CAD build for the part. Positions are in the model's coordinates, mm. A direction names the side the tool comes from. Round coordinates to 2 decimals unless told otherwise and drop trailing zeros. Loops run counter-clockwise (first coordinate to the right, second up) from the corner with the lowest first, then second, coordinate; pieces in that order, holes last.
Autodesk Inventor part; units mm, degrees
ref_plane "Work Plane1" through (-57.15, 3.175, 0) normal (1, 0, 0) x (0, 0, -1)
ref_plane "YZ Plane" through (0, 0, 0) normal (1, 0, 0) x (0, 1, 0)
ref_plane "XZ Plane" through (0, 0, 0) normal (0, 1, 0) x (-1, 0, 0)
sketch "Sketch1" plane through (0, 0, 0) normal (0, 0, 1) x (1, 0, 0)
  line L0 (0, 0) -> (-114.3, 0)
  line L1 (-114.3, 0) -> (-114.3, 63.5)
  line L2 (-114.3, 63.5) -> (0, 63.5)
  line L3 (0, 63.5) -> (0, 0)
  dimension "d7" = 114.3
  dimension "d8" = 63.5
extrude "Extrusion1" add sketch "Sketch1" along normal blind 6.35
sketch "Sketch2" plane through (0, 0, 6.35) normal (0, 0, 1) x (1, 0, 0)
  line L0 (0, 0) -> (0, 63.5)
  line L1 (-114.3, 63.5) -> (-114.3, 0)
  line L2 (-114.3, 0) -> (0, 0)
  line L3 (0, 63.5) -> (-114.3, 63.5)
sketch "Sketch3" plane through (0, 0, 6.35) normal (0, 0, 1) x (1, 0, 0)
  line L0 (-110.6716, 35.2666) -> (-52.0005, 35.2666) construction
  line L1 (-52.0005, 35.2666) -> (-52.0005, 28.3217) construction
  line L2 (-52.0005, 28.3217) -> (-110.6716, 28.3217) construction
  line L3 (-110.6716, 28.3217) -> (-110.6716, 35.2666) construction
  line L4 (-114.3, 63.5) -> (-114.3, 0)
  point P0 (0, 0)
extrude "Extrusion2" [suppressed]
fillet "Fillet2" radius 3.175 4 edges at (-114.3, 63.5, 3.175) (-114.3, 0, 3.175) (0, 0, 3.175) (0, 63.5, 3.175)
sketch "Sketch4" plane through (0, 0, 6.35) normal (0, 0, 1) x (1, 0, 0)
  point P0 (0, 0)
sketch "Sketch5" plane through (0, 0, 6.35) normal (0, 0, 1) x (1, 0, 0)
  point P0 (0, 0)
sketch "Sketch6" plane through (0, 0, 6.35) normal (0, 0, 1) x (1, 0, 0)
  point P0 (0, 0)
ref_plane "Work Plane1" through (-57.15, 3.175, 0) normal (1, 0, 0) x (0, 0, -1)
sketch "Sketch7" plane through (-111.125, 63.5, 0) normal (0, 1, 0) x (1, 0, 0)
  line L0 (107.95, -6.35) -> (0, -6.35)
  line L1 (107.95, 0) -> (0, 0)
  line L2 (0, -6.35) -> (0, -3.175)
  line L3 (0, -6.35) -> (0, 0)
  line L4 (0, 0) -> (0, -6.35)
  line L5 (0, -6.35) -> (0, -3.5306)
  line L6 (0, -3.5306) -> (6.985, -3.5306)
  line L7 (6.985, -3.5306) -> (11.8618, -3.5306)
  line L8 (11.8618, -3.5306) -> (11.8618, -1.651)
  line L9 (11.8618, -1.651) -> (6.985, -1.651)
  line L10 (6.985, -1.651) -> (6.985, -3.5306)
  point P0 (111.125, 0)
  dimension "d24" = 4.8768
  dimension "d25" = 1.8796
  dimension "d26" = 2.8194
  dimension "d27" = 6.985
extrude "Extrusion3" [suppressed]
sketch "Sketch8" plane through (-111.125, 0, 0) normal (0, -1, 0) x (1, 0, 0)
  line L0 (0, 0) -> (0, 6.35)
  line L1 (6.985, 3.5306) -> (6.985, 1.651)
  line L2 (11.8618, 1.651) -> (11.8618, 3.5306)
  line L3 (6.985, 1.651) -> (11.8618, 1.651)
  line L4 (11.8618, 1.651) -> (11.8618, 3.5306)
  line L5 (11.8618, 3.5306) -> (6.985, 3.5306)
  line L6 (6.985, 3.5306) -> (6.985, 1.651)
  line L7 (0, 0) -> (107.95, 0)
  point P0 (111.125, 0)
extrude "Extrusion4" [suppressed]
mirror "Mirror1" [suppressed]
mirror "Mirror2" [suppressed]
sketch "Sketch9" plane through (0, 0, 6.35) normal (0, 0, 1) x (1, 0, 0)
  point P0 (0, 0)
sketch "Sketch10" plane through (0, 0, 6.35) normal (0, 0, 1) x (1, 0, 0)
  line L0 (-111.2518, 27.0157) -> (-111.2518, 30.2464) construction
  line L1 (-111.2518, 30.2464) -> (-93.1484, 30.2464) construction
  line L2 (-93.1484, 30.2464) -> (-93.1484, 27.0157) construction
  line L3 (-93.1484, 27.0157) -> (-111.2518, 27.0157) construction
  line L4 (-114.3, 60.325) -> (-114.3, 3.175)
  line L5 (-114.3, 60.325) -> (-114.3, 3.175)
  line L6 (-114.3, 3.175) -> (-114.3, 31.75)
  line L7 (0, 3.175) -> (0, 60.325)
  line L8 (-88.3918, 11.8288) -> (-102.3042, 15.3115)
  line L9 (-102.3042, 15.3115) -> (-102.3042, 42.6731)
  line L10 (-102.3042, 42.6731) -> (-103.638, 42.988)
  spline S0 degree 2 poles (-103.638, 42.988) (-104.2308, 43.1362) (-105.2867, 42.8213) (-106.0833, 42.1173) (-106.5464, 41.0799) (-106.5464, 40.5242) knots 0 0 0 1 2 3 4 4 4
  line L11 (-106.5464, 40.5242) -> (-106.5464, 12.3845)
  spline S1 degree 2 poles (-106.5464, 12.3845) (-107.4912, 12.8106) (-109.7327, 13.8295) (-110.6775, 14.3297) knots 0 0 0 1 2 2 2
  line L12 (-110.6775, 14.3297) -> (-111.2518, 14.7743)
  line L13 (-111.2518, 14.7743) -> (-111.2518, 45.3222)
  spline S2 degree 2 poles (-111.2518, 45.3222) (-111.2518, 46.5078) (-110.6034, 49.1569) (-109.2881, 51.3984) (-107.38, 52.8434) (-106.0648, 52.8063) knots 0 0 0 1 2 3 4 4 4
  line L14 (-106.0648, 52.8063) -> (-88.3918, 48.3974)
  line L15 (-88.3918, 48.3974) -> (-88.3918, 39.1904)
  line L16 (-88.3918, 39.1904) -> (-97.5988, 41.469)
  line L17 (-97.5988, 41.469) -> (-97.5988, 23.3143)
  line L18 (-97.5988, 23.3143) -> (-88.3918, 21.0358)
  line L19 (-88.3918, 21.0358) -> (-88.3918, 11.8288)
  spline S3 degree 2 poles (-81.1464, 13.144) (-82.0912, 13.5701) (-84.3327, 14.589) (-85.2775, 15.0892) knots 0 0 0 1 2 2 2
  line L20 (-85.2775, 15.0892) -> (-85.8518, 15.5338)
  line L21 (-85.8518, 15.5338) -> (-85.8518, 54.3439)
  spline S4 degree 2 poles (-85.8518, 54.3439) (-84.907, 53.9734) (-82.6655, 52.9175) (-81.7207, 52.3803) knots 0 0 0 1 2 2 2
  line L22 (-81.7207, 52.3803) -> (-81.1464, 51.9357)
  line L23 (-81.1464, 51.9357) -> (-81.1464, 39.0051)
  line L24 (-81.1464, 39.0051) -> (-62.9918, 34.485)
  line L25 (-62.9918, 34.485) -> (-62.9918, 25.278)
  line L26 (-62.9918, 25.278) -> (-81.1464, 29.7981)
  line L27 (-81.1464, 29.7981) -> (-81.1464, 13.144)
  spline S5 degree 2 poles (-42.7788, 11.1619) (-41.4635, 11.1248) (-39.5555, 12.5512) (-38.2402, 14.7928) (-37.5918, 17.4419) (-37.5918, 18.6275) knots 0 0 0 1 2 3 4 4 4
  line L28 (-37.5918, 18.6275) -> (-37.5918, 46.6004)
  line L29 (-37.5918, 46.6004) -> (-60.4518, 52.2876)
  line L30 (-60.4518, 52.2876) -> (-60.4518, 43.0806)
  line L31 (-60.4518, 43.0806) -> (-42.2972, 38.5605)
  line L32 (-42.2972, 38.5605) -> (-42.2972, 23.407)
  spline S6 degree 2 poles (-42.2972, 23.407) (-42.2972, 22.8697) (-42.7603, 21.8509) (-43.5569, 21.1284) (-44.6128, 20.8134) (-45.1871, 20.9431) knots 0 0 0 1 2 3 4 4 4
  line L33 (-45.1871, 20.9431) -> (-60.4518, 24.7593)
  line L34 (-60.4518, 24.7593) -> (-60.4518, 15.5523)
  line L35 (-60.4518, 15.5523) -> (-42.7788, 11.1619)
  line L36 (-35.0518, 12.403) -> (-12.1918, 6.7158)
  line L37 (-12.1918, 6.7158) -> (-12.1918, 15.9228)
  line L38 (-12.1918, 15.9228) -> (-27.475, 19.7205)
  spline S7 degree 2 poles (-27.475, 19.7205) (-26.5302, 20.7393) (-24.1775, 22.9809) (-21.5655, 25.3336) (-18.8238, 27.6863) (-17.4715, 28.8534) knots 0 0 0 1 2 3 4 4 4
  line L39 (-17.4715, 28.8534) -> (-17.4715, 28.9645)
  spline S8 degree 2 poles (-17.4715, 28.9645) (-18.8238, 30.78) (-21.6026, 34.5406) (-24.2146, 38.1715) (-26.5302, 41.5986) (-27.475, 43.0992) knots 0 0 0 1 2 3 4 4 4
  line L40 (-27.475, 43.0992) -> (-12.1918, 39.283)
  line L41 (-12.1918, 39.283) -> (-12.1918, 48.49)
  line L42 (-12.1918, 48.49) -> (-35.0518, 54.1772)
  line L43 (-35.0518, 54.1772) -> (-35.0518, 44.2107)
  spline S9 degree 2 poles (-35.0518, 44.2107) (-34.5146, 43.0621) (-33.014, 40.376) (-31.2171, 37.5046) (-29.2164, 34.5406) (-28.1975, 33.0215) knots 0 0 0 1 2 3 4 4 4
  line L44 (-28.1975, 33.0215) -> (-27.0489, 31.2801)
  spline S10 degree 2 poles (-27.0489, 31.2801) (-29.9759, 28.4087) (-33.9959, 24.2221) (-35.0518, 22.3696) knots 0 0 0 1 2 2 2
  line L45 (-35.0518, 22.3696) -> (-35.0518, 12.403)
  point P0 (0, 0)
sketch "Sketch11" plane through (0, 3.175, 0) normal (1, 0, 0) x (0, 0, -1)
  line L0 (0, 0) -> (-6.35, 0)
  line L1 (-3.175, 0) -> (-3.175, 8.89)
  line L2 (-4.1148, 6.4516) -> (-2.2352, 6.4516)
  line L3 (-2.2352, 6.4516) -> (-2.2352, 11.3284)
  line L4 (-2.2352, 11.3284) -> (-4.1148, 11.3284)
  line L5 (-4.1148, 11.3284) -> (-4.1148, 6.4516)
  line L6 (-4.1148, 6.4516) -> (-2.2352, 11.3284) construction
  line L7 (-2.2352, 6.4516) -> (-4.1148, 11.3284) construction
  line L8 (0, 60.325) -> (-6.35, 60.325)
  line L9 (-3.175, 60.325) -> (-3.175, 47.625)
  line L10 (-4.1148, 45.1866) -> (-2.2352, 45.1866)
  line L11 (-2.2352, 45.1866) -> (-2.2352, 50.0634)
  line L12 (-2.2352, 50.0634) -> (-4.1148, 50.0634)
  line L13 (-4.1148, 50.0634) -> (-4.1148, 45.1866)
  line L14 (-4.1148, 45.1866) -> (-2.2352, 50.0634) construction
  line L15 (-2.2352, 45.1866) -> (-4.1148, 50.0634) construction
  point P0 (0, -3.175)
  point P1 (-2.2352, 47.625)
  dimension "d29" = 8.89
  dimension "d30" = 12.7
  dimension "d31" = 4.8768
  dimension "d32" = 1.8796
  dimension "d33" = 4.8768
  dimension "d34" = 1.8796
extrude "Extrusion5" cut sketch "Sketch11" against normal blind 9.652
extrude "Extrusion6" add sketch "Sketch10" along normal blind 1.5875
properties part number "custom  plate vertical"
Item 1: 3-axis set-ups, long thin cutter, end or side, ignore diameter. For faces 1 (the flat face through (-19.726, 17.795, 7.133)), 2 (the flat face through (-114.3, 31, 3)), 3 (the flat face through (-95.251, 13.546, 7.133)), 4 (the flat face through (0, 32, 3)), 5 (the flat face through (-5, 12, 4.115)): which of +Z, -Z, +X, -X, +Y, -Y reach the whole face in a straight line?
Answers follow:
face 1: +Z, +X
face 2: +Z, -Z, -X, +Y, -Y
face 3: +Z, -Y
face 4: +Z, -Z, +X, +Y, -Y
face 5: +X
Item 2: Flat gauge pins, fed straight in: P1, Ø0.5, axis at y = 17.5, z = 7, coming from the -X side; P2, Ø0.5, axis at y = 21, z = 7, coming from the +X side; P3, Ø0.6, axis at y = 12.5, z = 3, coming from the +X side. Where does each tip first touch, or does it go through?
Answers follow:
P1: stops at x = -111.25
P2: stops at x = -25.98
P3: stops at x = -9.65
Item 3: Cut at C-C, the plane x = -52.5. Give the cut face in (y, z), plus the area to 3 significant figures.
Answers follow:
outline: (0, 0) - (63.5, 0) - (63.5, 6.35) - (50.31, 6.35) - (50.31, 7.94) - (41.1, 7.94) - (41.1, 6.35) - (22.77, 6.35) - (22.77, 7.94) - (13.58, 7.94) - (13.58, 6.35) - (0, 6.35) - close
area: 432 mm2
Item 4: Probe line 1 (Z direction, x = -57.5, y = 34); line 2 (Y direction, x = -50, z = 7.25); line 3 (Y direction, x = -64, z = 7.25). List the from-to ranges inside material, lowest first.
Answers follow:
line 1: z = 0 to 6.35
line 2: y = 12.96 to 22.15, 40.48 to 49.69
line 3: y = 25.53 to 34.74
Item 5: Cut at B-B, the plane y = 55.5. Give the cut face in (x, z), plus the area to 3 significant figures.
Answers follow:
outline: (-114.3, 0) - (0, 0) - (0, 6.35) - (-114.3, 6.35) - close
area: 726 mm2
Item 6: Two-plate mould, pull along X, no slides. Class faces 6 (the cylindrical face through (-0.95, 0.91, 3.22)), 7 (the flat face through (-52.713, 22.824, 7.133)), 8 (the flat face through (-5, 51, 4.115)): released by +X, released by -X, zero draft, split by the parting line, or undercut.
Answers follow:
face 6: released by +X
face 7: undercut
face 8: zero draft
Item 7: Cut at A-A, the plane x = -72.5. Give the cut face in (y, z), plus the area to 3 significant figures.
Answers follow:
outline: (0, 0) - (63.5, 0) - (63.5, 6.35) - (36.85, 6.35) - (36.85, 7.94) - (27.65, 7.94) - (27.65, 6.35) - (0, 6.35) - close
area: 418 mm2
